The model under review builds one solid part; all positions refer to its coordinate system, in mm. A direction names the side the tool comes from. Give positions to 0.01 mm unless a question says otherwise; leave off trailing zeros. Order: outer loops, then holes, each group sorted by start corner. A loop starts at its lowest first (then second) coordinate and runs counter-clockwise, first axis right, second up. Notation, with made-up numbers: (21, -22) - (68, -22) arc R17 ccw to (68, -2) - close; hole circle Ø6 at (58, 66). An arc over 180 degrees is marked (long way). Answer as CSV lines item,"result". Start each with the question number.
from build123d import *

# Parameters (mm, degrees)
SKETCH_2_OUTSIDE_W  = 30.906
SKETCH_2_OUTSIDE_H  = 30.906
CUT_EXTRUDE_1_DEPTH = 25.070832973
SKETCH_3_OUTSIDE_W  = 114.288
SKETCH_3_OUTSIDE_H  = 116.188
SKETCH_3_OUTSIDE_R  = 9
CUT_EXTRUDE_2_DEPTH = 24.673878009
CUT_EXTRUDE_2_DRAFT = -60
SKETCH_4_OUTSIDE_W  = 28.814
SKETCH_4_OUTSIDE_H  = 30.714
SKETCH_4_OUTSIDE_R  = 8.75
CUT_EXTRUDE_3_DEPTH = 1.8


with BuildPart() as part:
    # Эскиз1 → Повернуть1 (revolve)
    with BuildSketch(Plane.XY, mode=Mode.PRIVATE) as revolve_1_sk:
        with BuildLine():
            Line((0, 3), (0, 7.5))
            Line((0, 7.5), (1, 8.5))
            Line((1, 8.5), (8, 8.5))
            Line((8, 8.5), (8, 10.45))
            Line((8, 10.45), (13, 10.45))
            Line((13, 10.45), (13, 7.6))
            ThreePointArc((13, 7.6), (13.219669914, 7.069669914), (13.75, 6.85))
            Line((13.75, 6.85), (15.889339828, 6.85))
            ThreePointArc((15.889339828, 6.85), (16.176352402, 6.907090351), (16.419669914, 7.069669914))
            Line((16.419669914, 7.069669914), (17.35, 8))
            Line((17.35, 8), (25.4, 8))
            Line((25.4, 8), (27, 6.4))
            Line((27, 6.4), (27, 5.25))
            Line((27, 5.25), (4, 5.25))
            ThreePointArc((4, 5.25), (3.292893219, 4.957106781), (3, 4.25))
            Line((3, 4.25), (3, 3))
            Line((3, 3), (0, 3))
        make_face()
    revolve(revolve_1_sk.sketch.rotate(Axis((0, 0, 0), (1, 0, 0)), 90), axis=Axis((0, 0, 0), (1, 0, 0)))

    # Эскиз2 outside → Вырез-Вытянуть1 (cut, through all)
    with BuildSketch(Plane.ZY.offset(-8)):
        Rectangle(SKETCH_2_OUTSIDE_W, SKETCH_2_OUTSIDE_H)
        Polygon((0, 10.969655115), (-9.5, 5.484827557), (-9.5, -5.484827557), (0, -10.969655115), (9.5, -5.484827557), (9.5, 5.484827557), align=None, mode=Mode.SUBTRACT)
    extrude(amount=-CUT_EXTRUDE_1_DEPTH, mode=Mode.SUBTRACT)


with BuildPart() as cut_extrude_2_tool:
    # Эскиз3 outside → Вырез-Вытянуть2 (with draft: the straight prism first)
    with BuildSketch(Plane.ZY.offset(-8)):
        Rectangle(SKETCH_3_OUTSIDE_W, SKETCH_3_OUTSIDE_H)
        Circle(SKETCH_3_OUTSIDE_R, mode=Mode.SUBTRACT)
    extrude(amount=-CUT_EXTRUDE_2_DEPTH)
    # Вырез-Вытянуть2: the draft: its side faces are tilted about the plane it starts from
    cut_extrude_2_sides = [cut_extrude_2_tool.faces().sort_by_distance(p)[0] for p in [
        (20.336939005, -58.094, 0),
        (20.336939005, 0, 57.144),
        (20.336939005, 58.094, 0),
        (20.336939005, 0, -57.144),
        (20.336939005, 0, -9),
    ]]
    draft(cut_extrude_2_sides, Plane.ZY.offset(-8), CUT_EXTRUDE_2_DRAFT)


with BuildPart() as part_1:
    add(part.part)

    # Вырез-Вытянуть2: cut by cut_extrude_2_tool
    add(cut_extrude_2_tool.part, mode=Mode.SUBTRACT)

    # Эскиз4 outside → Вырез-Вытянуть3 (cut)
    with BuildSketch(Plane(origin=(13, 0, 0), x_dir=(0, 0, -1), z_dir=(1, 0, 0))):
        Rectangle(SKETCH_4_OUTSIDE_W, SKETCH_4_OUTSIDE_H)
        Circle(SKETCH_4_OUTSIDE_R, mode=Mode.SUBTRACT)
    extrude(amount=-CUT_EXTRUDE_3_DEPTH, mode=Mode.SUBTRACT)


solid = part_1.part
Item 1: Clearance check with flat-ended pins moving along their axes: pin 1 (5 mm diameter, centred on y = 0, z = 0, fed in from +X); pin 2 (1 mm diameter, centred on x = 20, y = 4, fed in from +Z); pin 3 (4 mm diameter, centred on y = -6, z = 7.5, fed in from -X); pin 4 (1.5 mm diameter, centred on x = 9, z = 6, fed in from -Y). State where each tip first meets the part, or that it passes through.
Item 2: Mouldability with a two-part tool opening along Z and no side actions: class faces 1 (the face through (1.48, -0.9, 2.86)), 2 (the face through (4.549, -8.428, -1.107)), 3 (the face through (10, 0, -9.5)), 4 (the face through (9.7, 8.2, 4.8)) as released by +Z, released by -Z, zero draft, split by the parting line, or undercut.
Item 3: Take a section at B-B on x = 24.75. Write out the cut boundary in (y, z), and give its area (3 significant figures).
Item 4: For line 1 along Y through (x, z) = (18.5, 0); line 2 along Y through (x, z) = (2.3, 0); line 3 along Z through (x, y) = (10.75, 4.25), list the stretches that pass through material, from the lowest coordinate up.
Item 5: Machinability: for faces 5 (the face through (10.04, 5.24, 9.04)), 6 (the face through (21.43, 7.81, -1.73)), 7 (the face through (8, 3.3, -8)), which of the approach directions +Z, -Z, +X, -X, +Y, -Y give a long, thin tool a straight path to every point of the face, cutting with its end or side? Answer none if there is none.
Item 6: Take a section at A-A on x = 9.5. Write out the cut boundary in (y, z), and give its area (3 significant figures).
Data:
1,pin 1,"passes through"
1,pin 2,"stops at z = 7.19"
1,pin 3,"stops at x = 0.1"
1,pin 4,"stops at y = -7.94"
2,face 1,"undercut"
2,face 2,"split by the parting line"
2,face 3,"released by -Z"
2,face 4,"released by +Z"
3,outline,"circle Ø16 at (0, 0); hole circle Ø10.5 at (0, 0)"
3,area,"114 mm^2"
4,line 1,"y = -8 to -5.25, 5.25 to 8"
4,line 2,"y = -8.5 to -3, 3 to 8.5"
4,line 3,"z = -9.5 to -3.08, 3.08 to 9.5"
5,face 5,"+Z, +X, -X, +Y"
5,face 6,"+X"
5,face 7,"-X"
6,outline,"(-10.4, -0.98) - (-6.05, -8.52) arc R10.45 ccw to (-4.35, -9.5) - (4.35, -9.5) arc R10.45 ccw to (6.05, -8.52) - (10.4, -0.98) arc R10.45 ccw to (10.4, 0.98) - (6.05, 8.52) arc R10.45 ccw to (4.35, 9.5) - (-4.35, 9.5) arc R10.45 ccw to (-6.05, 8.52) - (-10.4, 0.98) arc R10.45 ccw to start; hole circle Ø10.5 at (0, 0)"
6,area,"223 mm^2"
